Could you check a few things on this model? Use its own coordinates, in mm. Face numbers are marked on the shaded views. A direction names the side the tool comes from. Round coordinates to 2 decimals unless told otherwise and drop trailing zeros. Loops run counter-clockwise (first coordinate to the right, second up) from the corner with the lowest first, then second, coordinate; pieces in that order, holes last. Notation, with made-up numbers: (-30.5, -38) -> (-14.5, -38) arc R13 ccw to (-14.5, -23) -> close; hole circle Ø2 at (-32, -35.5). An arc over 180 degrees is marked (long way). One line per item, written item: value.
Autodesk Inventor part; units mm, degrees
ref_plane "YZ Plane" through (0, 0, 0) normal (1, 0, 0) x (0, 1, 0)
ref_plane "XZ Plane" through (0, 0, 0) normal (0, 1, 0) x (-1, 0, 0)
ref_plane "XY Plane" through (0, 0, 0) normal (0, 0, 1) x (1, 0, 0)
sketch "Sketch1" plane through (0, 0, 0) normal (0, 0, 1) x (1, 0, 0)
  line L0 (-6.2155, 5.0202) -> (3.7845, 5.0202)
  line L1 (3.7845, 5.0202) -> (3.7845, 0.0202)
  line L2 (3.7845, 0.0202) -> (-6.2155, 0.0202)
  line L3 (-6.2155, 0.0202) -> (-6.2155, 5.0202)
  point P0 (0, 0)
  dimension "d0" = 10
  dimension "d1" = 5
extrude "Extrusion1" add sketch "Sketch1" along normal blind 15
sketch "Sketch2" plane through (0, 0, 15) normal (0, 0, 1) x (1, 0, 0)
  line L0 (-4.0285, 3.727) -> (1.9781, 3.727)
  line L1 (1.9781, 3.727) -> (1.9781, 1.58)
  line L2 (1.9781, 1.58) -> (-4.0285, 1.58)
  line L3 (-4.0285, 1.58) -> (-4.0285, 3.727)
  point P0 (0, 0)
extrude "Extrusion2" add sketch "Sketch2" along normal blind 1.5
chamfer "Chamfer1" distance 2.1 distance2 1.5 1 edges at (-1.0252, 3.727, 16.5) measured on face at (-2.0263, 3.0113, 16.5)
properties part number "cutter grp 17-1"
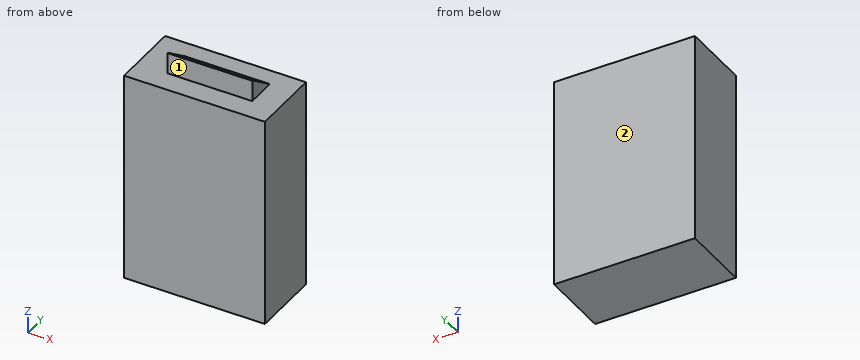
(1) If we section it at C-C, the plane z = 15.5: Please give me the cut outline in (x, y), then the cut area to 3 significant figures.
Recorded:
outline: (-4.03, 1.58) -> (1.98, 1.58) -> (1.98, 3.03) -> (-4.03, 3.03) -> close
area: 8.70 mm²
(2) If we section it at B-B, the plane y = 4: Please give me the cut outline in (x, z), then the cut area to 3 significant figures.
Recorded:
outline: (-6.22, 0) -> (3.78, 0) -> (3.78, 15) -> (-6.22, 15) -> close
area: 150 mm²
(3) For the marked faces 1 and 2, which set-ups out of +Z, -Z, +X, -X, +Y, -Y let a thin tool reach every point of the face, with its end or its side?
Recorded:
face 1: +Z, +X, -X, -Y
face 2: +Z, -Z, +X, -X, +Y
(4) If I drill on L1, parallel to Z at x = -3.5, y = 4.5; L2, parallel to Y at x = 1.25, z = 16.25; L3, parallel to Z at x = -1.25, y = 2.15, over which ranges is the centre line in solid material (lowest first)?
Recorded:
L1: 0 to 15
L2: 1.58 to 1.98
L3: 0 to 16.13
(5) If we section it at D-D, the plane y = 2.1: Please give me the cut outline in (x, z), then the cut area to 3 significant figures.
Recorded:
outline: (-6.22, 0) -> (3.78, 0) -> (3.78, 15) -> (1.98, 15) -> (1.98, 16.16) -> (-4.03, 16.16) -> (-4.03, 15) -> (-6.22, 15) -> close
area: 157 mm²
